Verification items for the finished model (mm, model axes). Coordinates: 2 decimals unless noted, no trailing zeros. Order: outer loops, then holes, each group sorted by start corner. A loop starts at its lowest first (then second) coordinate and runs counter-clockwise, first axis right, second up. Notation, with made-up numbers: M -7,7 L 4,7 A21 ccw 4,32 Z; hole C 27.5,37.5 d6. An arc over 180 degrees is marked long. Write item = value, one per line.
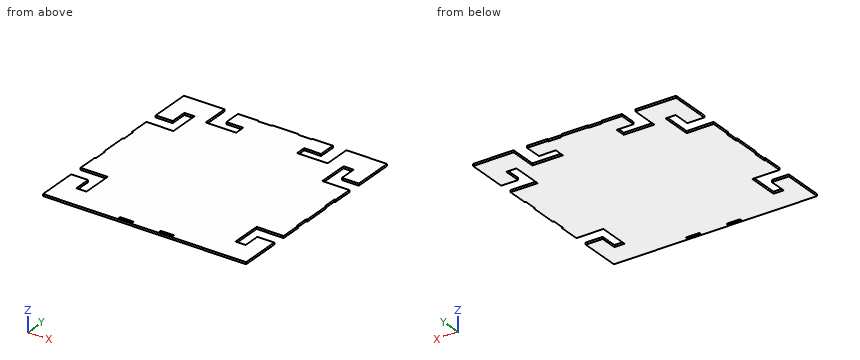
```python
from build123d import *

# Parameters (mm, degrees)
ESBO_O2_W                = 20
ESBO_O2_H                = 3
RESSALTO_EXTRUS_O1_DEPTH = 3


with BuildPart() as part:
    # Esboço2 → Ressalto-extrusão1 (new body)
    with BuildSketch(Plane.XY):
        Polygon((-63.645119203, -170), (-63.645119203, -110), (-38.645119203, -110), (-38.645119203, -135), (-23.645119203, -135), (-23.645119203, -90), (-63.645119203, -90), (-63.645119203, -60), (-62.145119203, -60), (-62.145119203, -40), (-63.645119203, -40), (-63.645119203, 0), (-62.145119203, 0), (-62.145119203, 20), (-63.645119203, 20), (-63.645119203, 50), (-23.645119203, 50), (-23.645119203, 95), (-38.645119203, 95), (-38.645119203, 70), (-63.645119203, 70), (-63.645119203, 130), (-3.645119203, 130), (-3.645119203, 90), (41.354880797, 90), (41.354880797, 105), (16.354880797, 105), (16.354880797, 130), (46.354880797, 130), (46.354880797, 128.5), (66.354880797, 128.5), (66.354880797, 130), (106.354880797, 130), (106.354880797, 128.5), (126.354880797, 128.5), (126.354880797, 130), (156.354880797, 130), (156.354880797, 105), (131.354880797, 105), (131.354880797, 90), (176.354880797, 90), (176.354880797, 130), (236.354880797, 130), (236.354880797, 70), (211.354880797, 70), (211.354880797, 95), (196.354880797, 95), (196.354880797, 50), (236.354880797, 50), (236.354880797, 20), (234.854880797, 20), (234.854880797, 0), (236.354880797, 0), (236.354880797, -40), (234.854880797, -40), (234.854880797, -60), (236.354880797, -60), (236.354880797, -90), (196.354880797, -90), (196.354880797, -135), (211.354880797, -135), (211.354880797, -110), (236.354880797, -110), (236.354880797, -170), align=None)
        with Locations((56.354880797, -166)):
            Rectangle(ESBO_O2_W, ESBO_O2_H, mode=Mode.SUBTRACT)
        with Locations((116.354880797, -166)):
            Rectangle(ESBO_O2_W, ESBO_O2_H, mode=Mode.SUBTRACT)
    extrude(amount=RESSALTO_EXTRUS_O1_DEPTH)


solid = part.part
```
Item 1: Gauge pin test, flat ends, axial feed: pin 1 (0.9 mm diameter, centred on x = 12, z = 1.5, fed in from +Y); pin 2 (0.9 mm diameter, centred on x = 61, z = 1, fed in from +Y). Record the tip position at first contact, or that the pin passes through.
Report:
pin_1 = 90
pin_2 = 128.5
Item 2: Scan lines: L1, parallel to Y at x = -31.5, z = 2.15; L2, parallel to X at y = 100.5, z = 2.7; L3, parallel to Y at x = 141, z = 1.2. Record each from-to range of solid material in increasing order. Write a range as from..to.
Report:
L1 = -170..-135, -90..50, 95..130
L2 = -63.65..-3.65, 41.35..131.35, 176.35..236.35
L3 = -170..90, 105..130
Item 3: Sectioned sample at B-B, the plane z = 0.9. Give the number of separate pieces and of enclosed holes in the cut face, then the cut area to 4 significant figures.
Report:
separate_pieces = 1
enclosed_holes = 2
area = 82,650 mm^2
Item 4: Sectioned sample at A-A, the plane y = -127. Enter the section's corners in (x, z), then the cut area to 3 significant figures.
Report:
outline = M -63.65,0 L -38.65,0 L -38.65,3 L -63.65,3 Z; M -23.65,0 L 196.35,0 L 196.35,3 L -23.65,3 Z; M 211.35,0 L 236.35,0 L 236.35,3 L 211.35,3 Z
area = 810 mm^2
